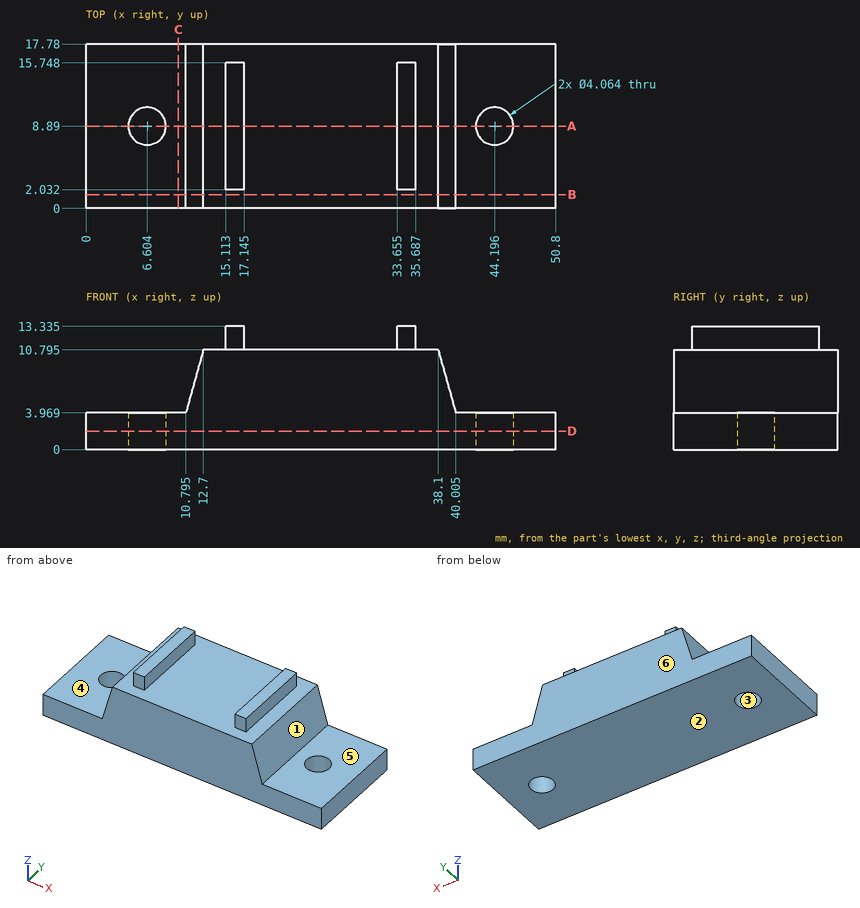
Answer from the drawing. Dimensions are ordinates in mm from the lowest x, y and z of the part. A direction names the side the tool comes from. Coordinates: 2 decimals unless noted, no trailing zeros. Loops run counter-clockwise (first coordinate to the right, second up) from the corner with the lowest first, then second, coordinate; pieces in that order, holes last. Notation, with made-up numbers: (-37, -36) -> (4, -36) arc R25 cw to (4, -15) -> close; hole circle Ø2 at (-9.5, 86.5). An arc over 180 degrees is marked (long way). Return JSON: item names as keys, results as strings.
Item 1: Find section C-C (x = 10). Determine the outline of the cut face in (y, z).
Answers:
{"outline": "(0, 0) -> (17.78, 0) -> (17.78, 3.97) -> (0, 3.97) -> close"}
Item 2: Find section A-A (y = 8.89). Determine the outline of the cut face in (x, z) (1 decimal), plus the area to 3 significant figures.
Answers:
{"outline": "(0, 0) -> (4.6, 0) -> (4.6, 4) -> (0, 4) -> close; (8.6, 0) -> (42.2, 0) -> (42.2, 4) -> (40, 4) -> (38.1, 10.8) -> (35.7, 10.8) -> (35.7, 13.3) -> (33.7, 13.3) -> (33.7, 10.8) -> (17.1, 10.8) -> (17.1, 13.3) -> (15.1, 13.3) -> (15.1, 10.8) -> (12.7, 10.8) -> (10.8, 4) -> (8.6, 4) -> close; (46.2, 0) -> (50.8, 0) -> (50.8, 4) -> (46.2, 4) -> close", "area": "366 mm2"}
Item 3: For the marked faces 4, 5 and 6, determine the directions among +Z, -Z, +X, -X, +Y, -Y from which every point of the face is accessible in a straight line to the end or side of a thin tool.
Answers:
{"face 4": "+Z, -X, +Y, -Y", "face 5": "+Z, +X, +Y, -Y", "face 6": "+Z, -Z, +X, -X, +Y"}
Item 4: Find the intervals of material crossed by probe 1 along X at (y, z) = (8.89, 1.55); probe 2 along X at (y, z) = (4.5, 12.5) (1 decimal); probe 3 along Z at (x, y) = (5.5, 16), in increasing order.
Answers:
{"probe 1": "x = 0 to 4.57, 8.64 to 42.16, 46.23 to 50.8", "probe 2": "x = 15.1 to 17.1, 33.7 to 35.7", "probe 3": "z = 0 to 3.97"}
Item 5: Find section B-B (y = 1.5). Determine the outline of the cut face in (x, z) (1 decimal).
Answers:
{"outline": "(0, 0) -> (50.8, 0) -> (50.8, 4) -> (40, 4) -> (38.1, 10.8) -> (12.7, 10.8) -> (10.8, 4) -> (0, 4) -> close"}
Item 6: For a pull along X with two mould halves and no side action, classify the marked faces 1, 2 and 3 as +X half, -X half, draft (parallel to the pull), parting line (faces both ways), or undercut.
Answers:
{"face 1": "+X half", "face 2": "draft", "face 3": "undercut"}
Item 7: Find section D-D (z = 2). Determine the outline of the cut face in (x, y).
Answers:
{"outline": "(0, 0) -> (50.8, 0) -> (50.8, 17.78) -> (0, 17.78) -> close; hole circle Ø4.06 at (6.6, 8.89); hole circle Ø4.06 at (44.2, 8.89)"}
Item 8: Flat-ended cylindrical pins translate along their axes: P1, Ø2, axis at x = 16.5, z = 12.5, coming from the -Y side; P2, Ø1.6, axis at x = 15.5, z = 12, coming from the +Y side; P3, Ø1, axis at x = 21, y = 2.5, coming from the +Z side (3 decimals). Find the tip coordinate at first contact, or state that the pin passes through.
Answers:
{"P1": "stops at y = 2.03", "P2": "stops at y = 15.75", "P3": "stops at z = 10.795"}
